For this review, use the dimensioned drawing (mm, ordinates from the lowest corner) and the shaded views. A direction names the side the tool comes from. Coordinates: 2 decimals unless noted, no trailing zeros. Loops run counter-clockwise (first coordinate to the right, second up) from the corner with the lowest first, then second, coordinate; pieces in that order, holes last. Notation, with made-up numbers: M -30,-23.5 L 24,-23.5 A15 ccw 24,-0.5 Z; hole C 66.5,73.5 d1. An arc over 180 degrees is marked long. Write item = value, one per line.
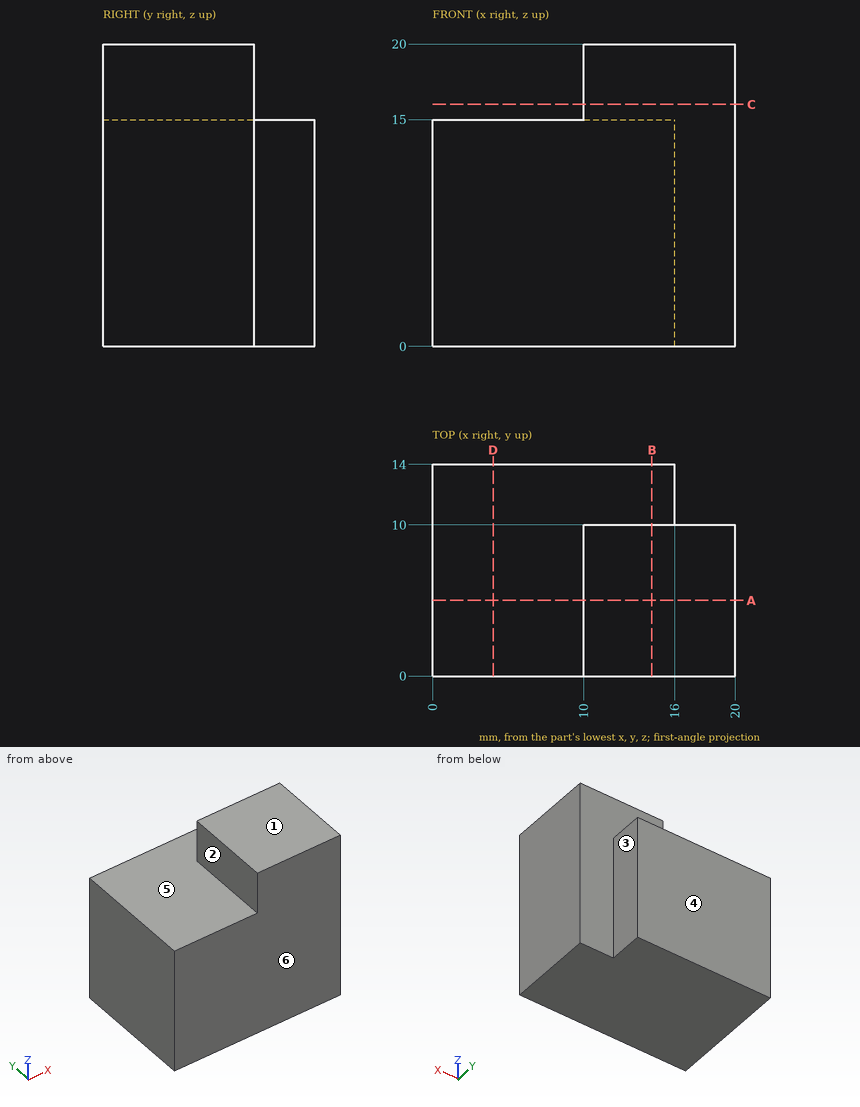
Q1. Add section D-D (x = 4). Write out the cut boundary in (y, z).
Solved:
outline = M 0,0 L 14,0 L 14,15 L 0,15 Z
Q2. Add section C-C (z = 16). Write out the cut boundary in (x, y), and give its area (3 significant figures).
Solved:
outline = M 10,0 L 20,0 L 20,10 L 10,10 Z
area = 100 mm²
Q3. For line 1 along Z through (x, y) = (8, 12.25); line 2 along Y through (x, z) = (19, 10); line 3 along X through (y, z) = (13, 13.5), list the stretches that pass through material, from the lowest coordinate up.
Solved:
line_1 = 0 to 15
line_2 = 0 to 10
line_3 = 0 to 16
Q4. Add section B-B (x = 14.5). Write out the cut boundary in (y, z).
Solved:
outline = M 0,0 L 14,0 L 14,15 L 10,15 L 10,20 L 0,20 Z
Q5. Draft analysis for pull direction Y (two halves, no side actions). For the marked faces 4, 5 and 6, state which applies: +Y half, -Y half, draft (parallel to the pull), parting line (faces both ways), or undercut.
Solved:
face_4 = +Y half
face_5 = draft
face_6 = -Y half
Q6. Machinability: for the marked faces 1, 2 and 3, which of the approach directions +Z, -Z, +X, -X, +Y, -Y give a long, thin tool a straight path to every point of the face, cutting with its end or side? Answer none if there is none.
Solved:
face_1 = +Z, +X, -X, +Y, -Y
face_2 = +Z, -X, +Y, -Y
face_3 = +Z, -Z, +X, +Y
Q7. For pin 1 Ø3 at (y, z) = (12, 11) entering from +X, flat-tipped, find the tip position at first contact; note if it passes through.
Solved:
pin_1 = 16
Q8. Add section A-A (y = 5). Write out the cut boundary in (x, z), and give its area (3 significant figures).
Solved:
outline = M 0,0 L 20,0 L 20,20 L 10,20 L 10,15 L 0,15 Z
area = 350 mm²
